Autodesk Inventor part; units mm, degrees
ref_plane "Work Plane1" through (-46.5, 0, 10) normal (-0.9659, 0, -0.2588) x (0, -1, 0)
ref_plane "Work Plane2" through (-46.5, 0, 10) normal (-0.8365, 0.5, -0.2241) x (0.2588, 0, -0.9659)
ref_plane "YZ Plane" through (0, 0, 0) normal (1, 0, 0) x (0, 1, 0)
sketch "Sketch1" plane through (0, 0, 0) normal (0, 0, 1) x (1, 0, 0)
  circle A0 centre (0, 0) radius 5
  circle A1 centre (0, 0) radius 8.45
  circle A2 centre (0, 0) radius 42.5
  circle A3 centre (0, 0) radius 45 construction
  circle A4 centre (-31.8198, 31.8198) radius 1.45
  arc A5 (-28.0933, 35.1535) -> (-35.1535, 28.0933) centre (-31.8198, 31.8198) ccw
  arc A6 (-35.1535, -28.0933) -> (-28.0933, -35.1535) centre (-31.8198, -31.8198) ccw
  circle A7 centre (-31.8198, -31.8198) radius 1.45
  arc A8 (28.0933, -35.1535) -> (35.1535, -28.0933) centre (31.8198, -31.8198) ccw
  circle A9 centre (31.8198, -31.8198) radius 1.45
  arc A10 (35.1535, 28.0933) -> (28.0933, 35.1535) centre (31.8198, 31.8198) ccw
  circle A11 centre (31.8198, 31.8198) radius 1.45
  line L0 (-31.8198, 31.8198) -> (31.8198, 31.8198) construction
  arc A12 (29.278, 36.1255) -> (-29.278, 36.1255) centre (0, 0) ccw
  arc A13 (-36.1255, 29.278) -> (-36.1255, -29.278) centre (0, 0) ccw
  arc A14 (-29.278, -36.1255) -> (29.278, -36.1255) centre (0, 0) ccw
  arc A15 (36.1255, -29.278) -> (36.1255, 29.278) centre (0, 0) ccw
  point P0 (0, -46.5)
  point P1 (0, 46.5)
  dimension "d2" = 10
  dimension "d3" = 16.9
  dimension "d4" = 85
  dimension "d5" = 90
  dimension "d6" = 2.9
  dimension "d7" = 5
  dimension "d8" = 360
  dimension "d24" = 93
extrude "Extrusion1" add sketch "Sketch1" against normal blind 3.75 contours A12 A10 A15 A8 A14 A6 A13 A5
extrude "Extrusion2" add sketch "Sketch1" along normal mid plane 7.5 contours A2
extrude "Extrusion3" add sketch "Sketch1" along normal blind 10 contours A12 A10 A15 A8 A14 A6 A13 A5
sketch "Sketch2" plane through (0, 0, 10) normal (0, 0, 1) x (1, 0, 0)
  arc A0 (-36.1255, 29.278) -> (-36.1255, -29.278) centre (0, 0) ccw
  line L0 (-46.5, 0) -> (-46.5, -31.8198) construction
  circle A1 centre (-31.8198, -31.8198) radius 1.45
ref_plane "Work Plane1" through (-46.5, 0, 10) normal (-0.9659, 0, -0.2588) x (0, -1, 0)
sketch "Sketch3" plane through (-46.5, 0, 10) normal (-0.9659, 0, -0.2588) x (0, -1, 0)
  line L0 (0, 0) -> (31.8198, 0)
  line L1 (0, 0) -> (0, -21.6943) construction
ref_plane "Work Plane2" through (-46.5, 0, 10) normal (-0.8365, 0.5, -0.2241) x (0.2588, 0, -0.9659)
sketch "Sketch4" plane through (-46.5, 0, 10) normal (-0.8365, 0.5, -0.2241) x (0.2588, 0, -0.9659)
  circle A0 centre (0, 0) radius 5.325
  point P0 (21.6943, -21.1637)
  point P1 (0, 0)
  dimension "d20" = 10.65
extrude "Extrusion5" cut sketch "Sketch4" along normal mid plane 20
sketch "Sketch5" plane through (0, 0, -3.75) normal (0, 0, -1) x (-1, 0, 0)
  circle A0 centre (0, 0) radius 5
  circle A1 centre (0, 0) radius 8.45
extrude "Extrusion6" add sketch "Sketch5" against normal blind 2.5
properties part number "Case Part 2"
Geometry: final body of the model. Coordinates: model frame, mm. A direction names the side the tool comes from. Round coordinates to 2 decimals unless told otherwise and drop trailing zeros. Write each loop counter-clockwise with the first axis right and the second up, starting at its lowest first coordinate (ties: lowest second). Pieces come first, ordered by that corner, then holes. Notation, with made-up numbers: M 33,-23 L 78,-23 A7 ccw 78,-14 Z; hole C 51,28 d2. An arc over 180 degrees is marked long. Answer in a Markdown table with one row per item. Add a question column.
(1) Ray query, L1, parallel to Y at x = 32, z = -0.25; L2, parallel to Z at x = 29, y = -17; L3, parallel to X at y = 18.5, z = 5.5. Return the intervals inside material, ascending.
(2) Reachability of faces 1 (the face through (1.08, -4.88, -2.52)), 2 (the face through (8.06, 2.54, 1.28)) from +Z, -Z, +X, -X, +Y, -Y: full face, straight path, thin tool, end or side. Return the list, or none.
(3) Cut plane D-D, the plane z = 1.75. Return the cut outline in (x, y).
(4) Cut plane B-B, the plane y = -18. Return the cut outline in (x, z).
(5) Cut plane C-C, the plane x = 18.5. Return the cut outline in (y, z).
(6) Draft query along X for faces 3 (the face through (-46.5, -0.4, 3)), 4 (the face through (-35.42, 35.29, 3.03)), 5 (the face through (35.29, 35.42, 3.03)), 6 (the face through (38, 21, 10)). Return one class per face: pulls with the +X half, pulls with the -X half, needs draft (parallel to the pull), parting line crosses it, or undercut.
(7) Cut plane A-A, the plane x = 0. Return the cut outline in (y, z), then the cut area to 3 significant figures.
(8) Contact query for flat-ended pins moving along their axis: pin 1 (1 mm diameter, centred on y = -12, z = 8, fed in from -X); pin 2 (16 mm diameter, centred on x = 0, y = 0, fed in from +Z); pin 3 (1 mm diameter, centred on x = -27, y = -3, fed in from +Z); pin 4 (2.5 mm diameter, centred on x = 31.82, y = -31.82, fed in from +Z). Output: stop coordinate, or through.
Established:
| question | item | result |
|---|---|---|
| 1 | L1 | -36.82 to -33.26, -30.38 to 30.38, 33.26 to 36.82 |
| 1 | L2 | -3.75 to 3.75 |
| 1 | L3 | -42.66 to -38.26, 38.26 to 42.66 |
| 2 | face 1 | +Z, -Z |
| 2 | face 2 | +Z |
| 3 | outline | M -36.13,-29.28 A5 ccw -29.28,-36.13 A46.5 ccw 29.28,-36.13 A5 ccw 36.13,-29.28 A46.5 ccw 36.13,29.28 A5 ccw 29.28,36.13 A46.5 ccw -29.28,36.13 A5 ccw -36.13,29.28 A46.5 ccw Z; hole C -31.82,-31.82 d2.9; hole C -31.82,31.82 d2.9; hole C 0,0 d16.9; hole C 31.82,-31.82 d2.9; hole C 31.82,31.82 d2.9 |
| 4 | outline | M -42.87,-3.75 L 42.87,-3.75 L 42.87,10 L 38.5,10 L 38.5,3.75 L -38.5,3.75 L -38.5,10 L -42.87,10 Z |
| 5 | outline | M -42.66,-3.75 L 42.66,-3.75 L 42.66,10 L 38.26,10 L 38.26,3.75 L -38.26,3.75 L -38.26,10 L -42.66,10 Z |
| 6 | face 3 | pulls with the -X half |
| 6 | face 4 | undercut |
| 6 | face 5 | undercut |
| 6 | face 6 | needs draft |
| 7 | outline | M -46.5,-3.75 L -5,-3.75 L -5,-1.25 L -8.45,-1.25 L -8.45,3.75 L -42.5,3.75 L -42.5,10 L -46.5,10 Z; M 5,-3.75 L 46.5,-3.75 L 46.5,10 L 42.5,10 L 42.5,3.75 L 8.45,3.75 L 8.45,-1.25 L 5,-1.25 Z |
| 7 | area | 638 mm² |
| 8 | pin 1 | x = -45.06 |
| 8 | pin 2 | z = -1.25 |
| 8 | pin 3 | z = 3.75 |
| 8 | pin 4 | through |
